Input: dimensioned drawing with shaded views. Units: mm. Origin: part minimum x, y, z. A direction names the side the tool comes from. Give positions to 0.01 mm unless a question says otherwise; leave off trailing zeros. Loops run counter-clockwise (first coordinate to the right, second up) from the corner with the lowest first, then second, coordinate; pieces in that order, holes last.
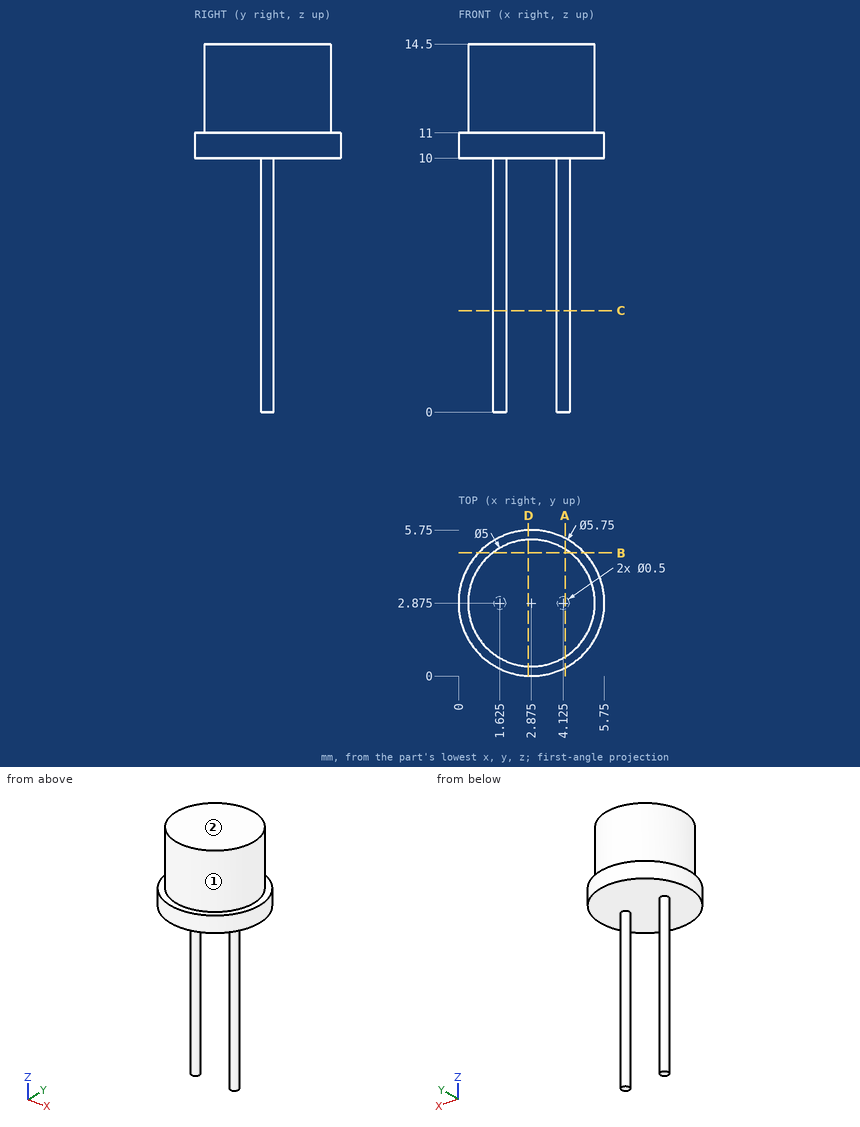
(1) Section A-A, the plane x = 4.2. Return the cut outline in (y, z) (3 decimals), then the cut area to 3 significant figures.
A:
outline: (0.324, 10) - (2.637, 10) - (2.637, 0) - (3.113, 0) - (3.113, 10) - (5.426, 10) - (5.426, 11) - (4.995, 11) - (4.995, 14.5) - (0.755, 14.5) - (0.755, 11) - (0.324, 11) - close
area: 24.7 mm2
(2) Section C-C, the plane z = 4. Return the cut outline in (x, y) (3 decimals).
A:
outline: circle Ø0.5 at (1.625, 2.875); circle Ø0.5 at (4.125, 2.875)
(3) Section B-B, the plane y = 4.85. Return the cut outline in (x, z), then the cut area to 3 significant figures.
A:
outline: (0.79, 10) - (4.96, 10) - (4.96, 11) - (4.41, 11) - (4.41, 14.5) - (1.34, 14.5) - (1.34, 11) - (0.79, 11) - close
area: 14.9 mm2
(4) Section D-D, the plane x = 2.75. Return the cut outline in (y, z), then the cut area to 3 significant figures.
A:
outline: (0, 10) - (5.75, 10) - (5.75, 11) - (5.37, 11) - (5.37, 14.5) - (0.38, 14.5) - (0.38, 11) - (0, 11) - close
area: 23.2 mm2
(5) Reachability of the marked faces 1 and 2 from +Z, -Z, +X, -X, +Y, -Y: full face, straight path, thin tool, end or side. Return the list, or none.
A:
face 1: +Z
face 2: +Z, +X, -X, +Y, -Y
(6) First-contact query: pin 1 (1.5 mm diameter, centred on x = 2.5, z = 12.5, fed in from -Y) (3 decimals); pin 2 (1.7 mm diameter, centred on x = 2, y = 2.5, fed in from -Z). Flat tips, straight axial feed; report the tip coordinate or a pass-through.
A:
pin 1: stops at y = 0.375
pin 2: stops at z = 0
(7) Ray query, line 1 along Z through (x, y) = (1.25, 3.75); line 2 along Z through (x, y) = (5.3, 4.2); line 3 along Y through (x, z) = (4.1, 1.5). Return the intervals inside material, ascending.
A:
line 1: z = 10 to 14.5
line 2: z = 10 to 11
line 3: y = 2.63 to 3.12
